from build123d import *

# Parameters (mm, degrees)
F0_W     = 76
F0_H     = 23
F1_DEPTH = 8
F3_DEPTH = 70
F4_R     = 2.5
F5_DEPTH = 25


with BuildPart() as f1:
    # F0 (on Top) → F1 (new body)
    with BuildSketch(Plane.XY):
        with Locations((-1.670267, -10.164521)):
            Rectangle(F0_W, F0_H)
    extrude(amount=F1_DEPTH)

    # F2 (on face) → F3 (join)
    with BuildSketch(Plane.XY.offset(8)):
        Polygon((-39.670267, 1.335479), (-39.670267, -21.664521), (-32.670267, -21.664521), (-32.670267, -18.664521), (-36.670267, -18.664521), (-36.670267, -8.664521), (-32.670267, -8.664521), (-32.670267, -3.664521), (29.329733, -3.664521), (29.329733, -8.664521), (33.329733, -8.664521), (33.329733, -18.664521), (29.329733, -18.664521), (29.329733, -21.664521), (36.329733, -21.664521), (36.329733, 1.335479), align=None)
    extrude(amount=F3_DEPTH)

    # F4 (on face) → F5 (cut)
    with BuildSketch(Plane.XZ.offset(3.664521)):
        with Locations((17.329733, 56)):
            Circle(F4_R)
        with Locations((-20.670267, 56)):
            Circle(F4_R)
        with Locations((-20.670267, 26)):
            Circle(F4_R)
        with Locations((17.329733, 26)):
            Circle(F4_R)
    extrude(amount=-F5_DEPTH, mode=Mode.SUBTRACT)


solid = f1.part
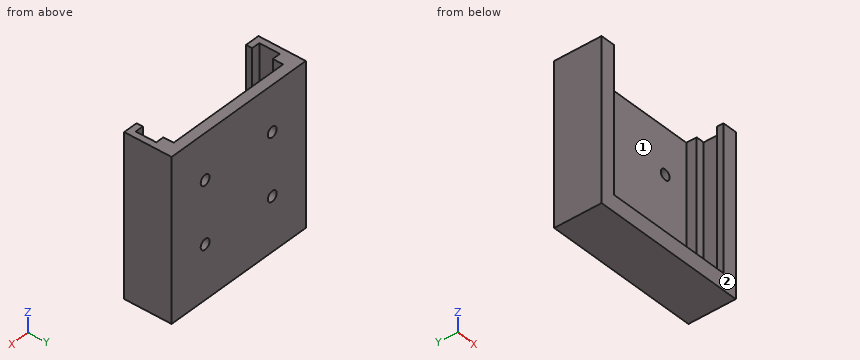
Here's how the part is built. I have some questions about the finished solid (model axes, mm). Face numbers are marked on the shaded views. A direction names the side the tool comes from. Coordinates: 2 decimals unless noted, no trailing zeros. Order: outer loops, then holes, each group sorted by start corner. A loop starts at its lowest first (then second) coordinate and runs counter-clockwise, first axis right, second up.
Item 1: If we section it at D-D on z = 47: List the corners of the cut face in (x, y) for me, plus the area to 3 significant figures.
Result sheet:
outline: (-39.67, -21.66) - (-32.67, -21.66) - (-32.67, -18.66) - (-36.67, -18.66) - (-36.67, -8.66) - (-32.67, -8.66) - (-32.67, -3.66) - (29.33, -3.66) - (29.33, -8.66) - (33.33, -8.66) - (33.33, -18.66) - (29.33, -18.66) - (29.33, -21.66) - (36.33, -21.66) - (36.33, 1.34) - (-39.67, 1.34) - close
area: 552 mm2
Item 2: If we section it at C-C on x = 11.5: List the corners of the cut face in (y, z) for me, plus the area to 3 significant figures.
Result sheet:
outline: (-21.66, 0) - (1.34, 0) - (1.34, 78) - (-3.66, 78) - (-3.66, 8) - (-21.66, 8) - close
area: 534 mm2
Item 3: For P1, Ø3, axis at x = -26.5, y = -11, coming from the +Z side; P2, Ø6, axis at x = 11.5, z = 27.5, coming from the -Y side, each with a flat end and sliding along its axis, tell me the tip position at first contact or that it passes through.
Result sheet:
P1: stops at z = 8
P2: stops at y = -3.66
Item 4: For the marked faces 1 and 2, which set-ups out of +Z, -Z, +X, -X, +Y, -Y let a thin tool reach every point of the face, with its end or its side?
Result sheet:
face 1: +Z, -Y
face 2: +Z, -Z, +X, -X, -Y
Item 5: I need wall thicknesses on line 1 (X direction, y = -11.5, z = 31); line 2 (X direction, y = -7.75, z = 27.5); line 3 (Z direction, x = 27, y = -6.25). Which ranges of each line are inside material? Lowest first, please.
Result sheet:
line 1: x = -39.67 to -36.67, 33.33 to 36.33
line 2: x = -39.67 to -32.67, 29.33 to 36.33
line 3: z = 0 to 8
Item 6: If we section it at B-B on y = -15.5: List the corners of the cut face in (x, z) for me.
Result sheet:
outline: (-39.67, 0) - (36.33, 0) - (36.33, 78) - (33.33, 78) - (33.33, 8) - (-36.67, 8) - (-36.67, 78) - (-39.67, 78) - close
Item 7: If we section it at A-A on z = 56: List the corners of the cut face in (x, y) for me, plus the area to 3 significant figures.
Result sheet:
outline: (-39.67, -21.66) - (-32.67, -21.66) - (-32.67, -18.66) - (-36.67, -18.66) - (-36.67, -8.66) - (-32.67, -8.66) - (-32.67, -3.66) - (-23.17, -3.66) - (-23.17, 1.34) - (-39.67, 1.34) - close; (-18.17, -3.66) - (14.83, -3.66) - (14.83, 1.34) - (-18.17, 1.34) - close; (19.83, -3.66) - (29.33, -3.66) - (29.33, -8.66) - (33.33, -8.66) - (33.33, -18.66) - (29.33, -18.66) - (29.33, -21.66) - (36.33, -21.66) - (36.33, 1.34) - (19.83, 1.34) - close
area: 502 mm2
